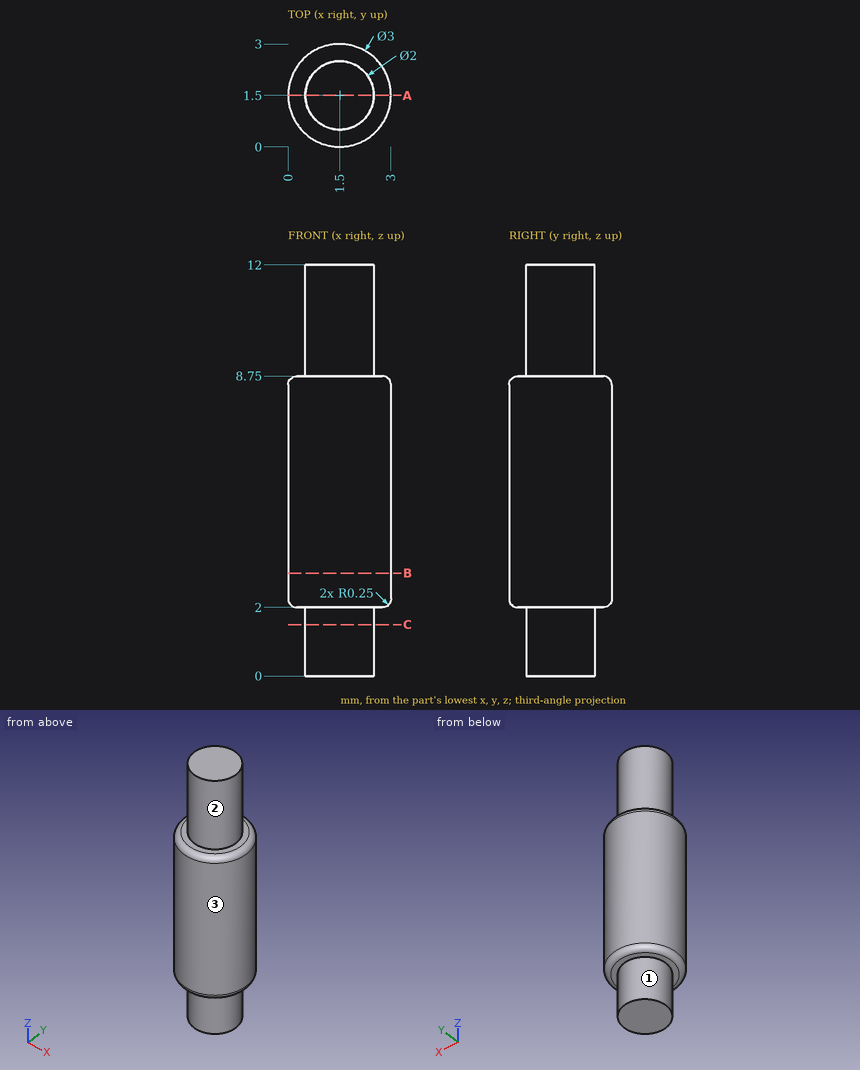
Geometry check sheet. Reference: drawing and pictorial views, mm from the part's lowest x, y, z. A direction names the side the tool comes from. Round coordinates to 2 decimals unless told otherwise and drop trailing zeros. Loops run counter-clockwise (first coordinate to the right, second up) from the corner with the lowest first, then second, coordinate; pieces in that order, holes last. Notation, with made-up numbers: (46, -4.5) -> (65, -4.5) arc R23 cw to (65, 23.5) -> close; hole circle Ø7 at (70, 46). An arc over 180 degrees is marked (long way). Answer as a JSON object with one key per item and string values. Group by question number.
Item 1: Thickness scan on line 1 along Z through (x, y) = (0.65, 0.65); line 2 along X through (y, z) = (2.1, 5.5). Record the ranges inside material, lowest first.
Item 2: Cross-section at A-A, the plane y = 1.5. Record the cut outline in (x, z).
Item 3: Set-up check for the marked faces 1, 2 and 3: record each of +Z, -Z, +X, -X, +Y, -Y from which the full face is reachable in a straight line by a thin tool's end or side.
Item 4: Cross-section at C-C, the plane z = 1.5. Record the cut outline in (x, y).
Item 5: Depth check by flat-ended pin: pin 1 Ø1.5 at (y, z) = (0.5, 2) entering from +X; pin 2 Ø1 at (y, z) = (2, 10.5) entering from +X. Enter the tip coordinate at first touch or a pass-through.
Item 6: Cross-section at B-B, the plane z = 3. Record the cut outline in (x, y), plus the area to 3 significant figures.
Determined:
{
 "1": {"line 1": "z = 2 to 8.75", "line 2": "x = 0.13 to 2.87"},
 "2": {"outline": "(0, 2.25) arc R0.25 ccw to (0.25, 2) -> (0.5, 2) -> (0.5, 0) -> (2.5, 0) -> (2.5, 2) -> (2.75, 2) arc R0.25 ccw to (3, 2.25) -> (3, 8.5) arc R0.25 ccw to (2.75, 8.75) -> (2.5, 8.75) -> (2.5, 12) -> (0.5, 12) -> (0.5, 8.75) -> (0.25, 8.75) arc R0.25 ccw to (0, 8.5) -> close"},
 "3": {"face 1": "-Z", "face 2": "+Z", "face 3": "+Z, -Z"},
 "4": {"outline": "circle Ø2 at (1.5, 1.5)"},
 "5": {"pin 1": "stops at x = 2.97", "pin 2": "stops at x = 2.5"},
 "6": {"outline": "circle Ø3 at (1.5, 1.5)", "area": "7.07 mm²"}
}
